```python
from build123d import *

# Parameters (mm, degrees)
EXTRUDE_1_DEPTH             = 104
EXTRUDE_1_2_DEPTH           = 61
EXTRUDE_1_2_DEPTH_BACK      = 61
EXTRUDE_5_DEPTH             = 69.333333333
CUT_EXTRUDE_5_DEPTH         = 320.954684291
CUT_EXTRUDE_5_DEPTH_BACK    = 320.954684291
SKETCH_13_OUTSIDE_W         = 481.25
SKETCH_13_OUTSIDE_H         = 210.25
RIB_START                   = -2.5
RIB_2_DEPTH                 = 5
FILLET_1_R                  = 10
EXTRUDE_7_REACH             = 315.142
EXTRUDE_7_DIRECTION_2_REACH = 315.142
CUT_EXTRUDE_3_DEPTH         = 314.142140249
CUT_EXTRUDE_3_DEPTH_BACK    = 314.142140249
SKETCH_10_R                 = 5
EXTRUDE_8_DEPTH             = 98
CUT_EXTRUDE_6_DEPTH         = 323.308858085


# Read off the part's stored shape, not the designer's step: 보강대2
with BuildPart() as part:
    # 스케치1 → Extrude 1 (new body)
    with BuildSketch(Plane(origin=(0, 0, 0), x_dir=(1, 0, 0), z_dir=(0, 1, 0))):
        Polygon((0, 61), (0, -61), (-104, 0), align=None)
        Polygon((-10, 43.541395957), (-84.234511141, 0), (-10, -43.541395957), align=None, mode=Mode.SUBTRACT)
    extrude(amount=EXTRUDE_1_DEPTH)


with BuildPart() as body_2:
    # 스케치3 → Extrude 1 2 (new, two sides: drawn at the far end of the back side and taken through both)
    with BuildSketch(Plane.XY.offset(-EXTRUDE_1_2_DEPTH_BACK)):
        Polygon((0, 0), (50, 0), (91.711375741, 35), (148.654022129, 35), (199, -25), (244, -25), (244, -19), (201.797845949, -19), (151.451868078, 41), (89.527554335, 41), (47.816178594, 6), (0, 6), align=None)
    extrude(amount=EXTRUDE_1_2_DEPTH + EXTRUDE_1_2_DEPTH_BACK)

    # 스케치13 outside → 컷-돌출5 (cut, two sides: drawn at the far end of the back side and taken through both)
    with BuildSketch(Plane(origin=(0, -19, 0), x_dir=(1, 0, 0), z_dir=(0, 1, 0)).offset(-CUT_EXTRUDE_5_DEPTH_BACK)):
        with Locations((92.5, 0)):
            Rectangle(SKETCH_13_OUTSIDE_W, SKETCH_13_OUTSIDE_H)
        Polygon((0, 61), (244, 30), (244, -30), (0, -61), align=None, mode=Mode.SUBTRACT)
    extrude(amount=CUT_EXTRUDE_5_DEPTH + CUT_EXTRUDE_5_DEPTH_BACK, mode=Mode.SUBTRACT)


with BuildPart() as body_3:
    # 스케치12 → 보스-돌출5 (new body)
    with BuildSketch(Plane.XZ.offset(25)):
        Polygon((244, 30), (244, -30), (289, 0), align=None)
        Polygon((254, 11.314829082), (270.972243623, 0), (254, -11.314829082), align=None, mode=Mode.SUBTRACT)
    extrude(amount=-EXTRUDE_5_DEPTH)


with BuildPart() as part_1:
    add(part.part)

    # Combine 1: union body 3, body 2
    add(body_3.part)
    add(body_2.part)

    # 보강대2 outline → 보강대2 (add)
    with BuildSketch(Plane.XY.offset(RIB_START)):
        Polygon((231.330664299, 44.333333333), (181.264386305, 104), (0, 104), (0, 6), (47.816178594, 6), (89.527554335, 41), (151.451868078, 41), (201.797845949, -19), (244, -19), (244, 44.333333333), align=None)
    extrude(amount=RIB_2_DEPTH)

    # 필렛1
    fillet_1_edges = [part_1.edges().sort_by_distance(p)[0] for p in [
        (181.264386305, 104, 0),
        (199, -25, 0),
        (201.797845949, -19, 18.93087454),
        (151.451868078, 41, 22.129082151),
        (89.527554335, 41, 26.062798802),
        (47.816178594, 6, 28.712496852),
        (50, 0, 0),
        (91.711375741, 35, 0),
        (148.654022129, 35, 0),
        (47.816178594, 6, -28.712496852),
        (89.527554335, 41, -26.062798802),
        (151.451868078, 41, -22.129082151),
        (201.797845949, -19, -18.93087454),
        (231.330664299, 44.333333333, 0),
    ]]
    fillet(fillet_1_edges, radius=FILLET_1_R)

    # 보스-돌출7: up to this plane
    extrude_7_end = Plane(origin=(244, -25, 30), z_dir=(0.12603604726758494, 0, 0.9920256623642169))
    # 스케치9 → 보스-돌출7 (add, up to the surface)
    with BuildSketch(Plane.XY, mode=Mode.PRIVATE) as extrude_7_sk1:
        with BuildLine():
            Line((244, -19), (219, -19))
            Line((219, -19), (219, -15))
            ThreePointArc((219, -15), (221.928932188, -7.928932188), (229, -5))
            Line((229, -5), (244, -5))
            Line((244, -5), (244, -19))
        make_face()
    extrude_7_tool1 = split(extrude(extrude_7_sk1.sketch, amount=EXTRUDE_7_REACH, mode=Mode.PRIVATE), bisect_by=extrude_7_end, keep=Keep.BOTH, mode=Mode.PRIVATE)
    add(extrude_7_tool1.solids().sort_by_distance((232.170595, -12.311336, 0))[0])

    # 보스-돌출7 direction 2: up to this plane
    extrude_7_direction_2_end = Plane(origin=(0, -25, -61), z_dir=(0.12603604726758494, 0, -0.9920256623642169))
    # 스케치9 → 보스-돌출7 direction 2 (add, up to the surface)
    with BuildSketch(Plane.XY, mode=Mode.PRIVATE) as extrude_7_direction_2_sk1:
        with BuildLine():
            Line((244, -19), (219, -19))
            Line((219, -19), (219, -15))
            ThreePointArc((219, -15), (221.928932188, -7.928932188), (229, -5))
            Line((229, -5), (244, -5))
            Line((244, -5), (244, -19))
        make_face()
    extrude_7_direction_2_tool1 = split(extrude(extrude_7_direction_2_sk1.sketch, amount=-EXTRUDE_7_DIRECTION_2_REACH, mode=Mode.PRIVATE), bisect_by=extrude_7_direction_2_end, keep=Keep.BOTH, mode=Mode.PRIVATE)
    add(extrude_7_direction_2_tool1.solids().sort_by_distance((232.170595, -12.311336, 0))[0])

    # 스케치10 → 컷-돌출3 (cut, two sides: drawn at the far end of the back side and taken through both)
    with BuildSketch(Plane.XY.offset(-CUT_EXTRUDE_3_DEPTH_BACK)):
        with Locations((229, -15)):
            Circle(SKETCH_10_R)
    extrude(amount=CUT_EXTRUDE_3_DEPTH + CUT_EXTRUDE_3_DEPTH_BACK, mode=Mode.SUBTRACT)

    # 스케치14 → 보스-돌출8 (add)
    with BuildSketch(Plane(origin=(0, 104, 0), x_dir=(1, 0, 0), z_dir=(0, 1, 0))):
        with BuildLine():
            Line((-10, -20), (-10, -10))
            ThreePointArc((-10, -10), (0, 0), (-10, 10))
            Line((-10, 10), (-10, 20))
            ThreePointArc((-10, 20), (10, 0), (-10, -20))
        make_face()
    extrude(amount=-EXTRUDE_8_DEPTH)

    # 스케치14<2> → 컷-돌출6 (cut, through all)
    with BuildSketch(Plane(origin=(0, 104, 0), x_dir=(1, 0, 0), z_dir=(0, 1, 0))):
        with BuildLine():
            Line((-10, 10), (-10, -10))
            ThreePointArc((-10, -10), (0, 0), (-10, 10))
        make_face()
    extrude(amount=-CUT_EXTRUDE_6_DEPTH, mode=Mode.SUBTRACT)


solid = part_1.part
```
Could you check a few things on this model? Use its own coordinates, in mm. A direction names the side the tool comes from. Coordinates: 2 decimals unless noted, no trailing zeros. Write each loop counter-clockwise with the first axis right and the second up, starting at its lowest first coordinate (ties: lowest second). Pieces come first, ordered by that corner, then holes. Notation, with made-up numbers: (-37, -34) - (-18, -34) arc R23 ccw to (-18, -14) - close; hole circle Ø3 at (38, 19.25). An arc over 180 degrees is marked (long way). Use a Markdown table: item, result.
Q1. Imagine slicing it at A-A (x = -18.5). List the corners of the cut face in (y, z) for me.
Geometry check:
| item | result |
|---|---|
| outline | (0, -50.15) - (104, -50.15) - (104, -38.56) - (0, -38.56) - close; (0, 38.56) - (104, 38.56) - (104, 50.15) - (0, 50.15) - close |
Q2. Imagine slicing it at B-B (x = 25.5). List the corners of the cut face in (y, z) for me.
Geometry check:
| item | result |
|---|---|
| outline | (0, -57.76) - (6, -57.76) - (6, -2.5) - (104, -2.5) - (104, 2.5) - (6, 2.5) - (6, 57.76) - (0, 57.76) - close |
Q3. I'm going to push flat-ended pins straight in: pin 1 Ø10 at (x, y) = (34.5, 41.5) entering from -Z; pin 2 Ø3 at (y, z) = (-16.5, 18) entering from -X; pin 3 Ø10 at (x, z) = (14, 6) entering from -Y. Where does each tip first touch, or does it pass through?
Geometry check:
| item | result |
|---|---|
| pin 1 | stops at z = -2.5 |
| pin 2 | stops at x = 190.61 |
| pin 3 | stops at y = 0 |
Q4. Thinking about a two-plate mould opening in Z: for faces 1 (the cylindrical face through (0, 53, 0)), 2 (the flat face through (22, 6, 31)), 3 (the flat face through (266.2, 9.2, -15.2)), 4 (the flat face through (130.468, 37.487, 44.424)), which applies, +Z half, -Z half, draft (parallel to the pull), parting line (faces both ways), or undercut?
Geometry check:
| item | result |
|---|---|
| face 1 | undercut |
| face 2 | draft |
| face 3 | -Z half |
| face 4 | +Z half |
Q5. Please list where these lines run through material, in increasing order: L1, parallel to Y at x = 229, z = 12.5; L2, parallel to X at y = -15, z = 3; L3, parallel to X at y = -15, z = -13.
Geometry check:
| item | result |
|---|---|
| L1 | y = -25 to -20, -10 to -5 |
| L2 | x = 190.61 to 198.44, 219 to 224, 234 to 254, 266.47 to 284.5 |
| L3 | x = 190.61 to 198.44, 219 to 224, 234 to 269.5 |
Q6. Which directions (+Z, -Z, +X, -X, +Y, -Y) give clear straight access to the entire face, cutting with the end or side of a thin tool? Please do faces 5 (the flat face through (-47.637, 51.272, 21.466)), 6 (the flat face through (236, -5, -17)), 7 (the cylindrical face through (148.16, 34.09, 0.6)), 8 (the cylindrical face through (150.96, 40.09, 22.7)).
Geometry check:
| item | result |
|---|---|
| face 5 | +Y, -Y |
| face 6 | -Z, +Y |
| face 7 | +Z, -Z, -Y |
| face 8 | +Z, +Y |
